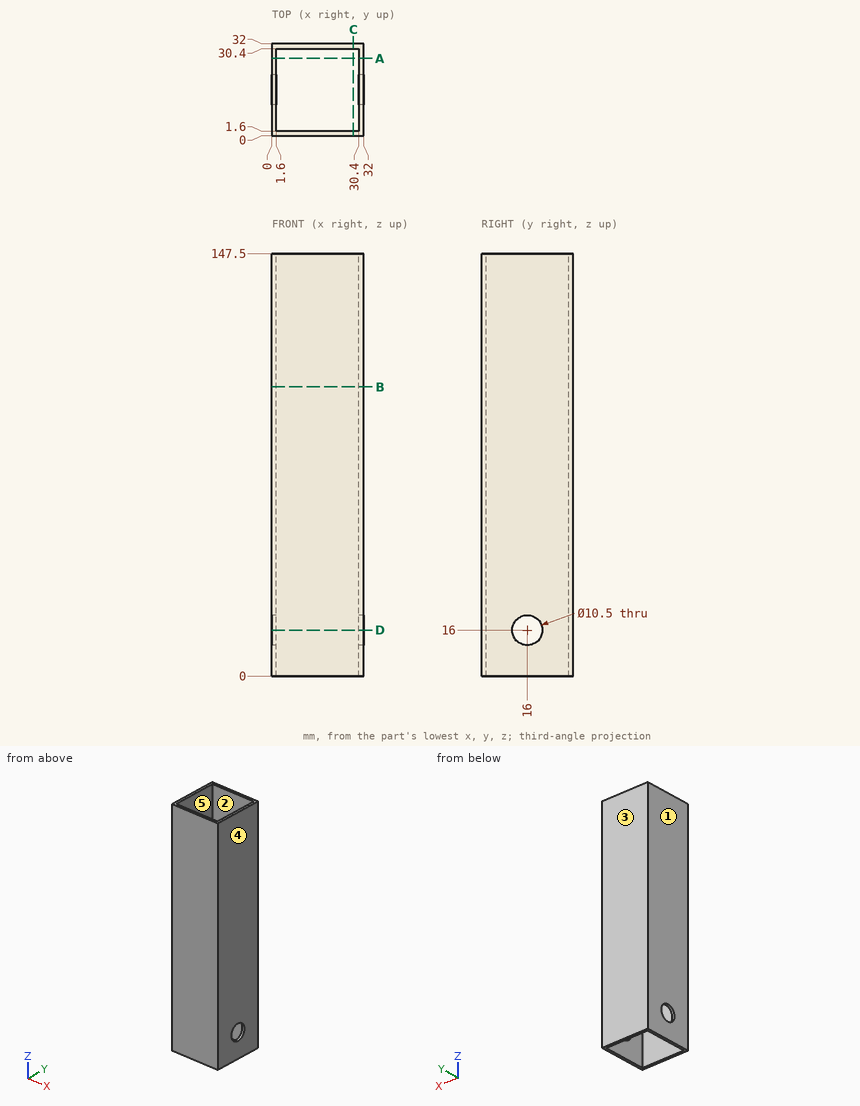
Geometry check sheet. Reference: drawing and pictorial views, mm from the part's lowest x, y, z. A direction names the side the tool comes from. Give positions to 0.01 mm unless a question says otherwise; leave off trailing zeros. Write each loop counter-clockwise with the first axis right and the second up, starting at its lowest first coordinate (ties: lowest second). Pieces come first, ordered by that corner, then holes. Notation, with made-up numbers: M -20.75,7.5 L 8.25,7.5 A22 cw 8.25,26.5 Z; hole C 52,-28.75 d5. An arc over 180 degrees is marked long. Put each result on its own line as item: value. Start each with the question number.
1. Section check B-B (z = 101). Record the cut outline in (x, y), and give its area (3 significant figures).
2. Section check A-A (y = 27). Record the cut outline in (x, z), and give its area (3 significant figures).
3. Go/stop test with flat-tipped pins: pin 1 Ø4 at (y, z) = (27, 49) entering from -X; pin 2 Ø5 at (x, y) = (13, 6.5) entering from -Z. Record where each tip stops, or that it passes through.
4. Scan lines: line 1 along Z through (x, y) = (31, 16); line 2 along X through (y, z) = (22, 96). Record each from-to range of solid material in increasing order. Write a range as [from, to].
5. Section check D-D (z = 16). Record the cut outline in (x, y).
6. Set-up check for the marked faces 1 and 2: record each of +Z, -Z, +X, -X, +Y, -Y from which the full face is reachable in a straight line by a thin tool's end or side.
7. Draft check along X on the marked faces 3, 4 and 5. Enter one of: +X half, -X half, draft (parallel to the pull), parting line (faces both ways), or undercut.
Answer list:
1. outline: M 0,0 L 32,0 L 32,32 L 0,32 Z; hole M 1.6,1.6 L 30.4,1.6 L 30.4,30.4 L 1.6,30.4 Z
1. area: 195 mm2
2. outline: M 0,0 L 1.6,0 L 1.6,147.5 L 0,147.5 Z; M 30.4,0 L 32,0 L 32,147.5 L 30.4,147.5 Z
2. area: 472 mm2
3. pin 1: x = 0
3. pin 2: through
4. line 1: [0, 10.75], [21.25, 147.5]
4. line 2: [0, 1.6], [30.4, 32]
5. outline: M 0,0 L 32,0 L 32,10.75 L 30.4,10.75 L 30.4,1.6 L 1.6,1.6 L 1.6,10.75 L 0,10.75 Z; M 0,21.25 L 1.6,21.25 L 1.6,30.4 L 30.4,30.4 L 30.4,21.25 L 32,21.25 L 32,32 L 0,32 Z
6. face 1: +Z, -Z, -X, +Y, -Y
6. face 2: +Z, -Z
7. face 3: draft
7. face 4: +X half
7. face 5: undercut
